For this review, take the finished solid that the model builds, in its own axes (mm). A direction names the side the tool comes from. Round coordinates to 2 decimals unless told otherwise and drop trailing zeros. Loops run counter-clockwise (first coordinate to the right, second up) from the corner with the lowest first, then second, coordinate; pieces in that order, holes last.
1. Consider section B-B on z = 43.5. State the section outline as (x, y) points.
2. Tool access review of faces 5 (the flat face through (-46, 29, -11)), 6 (the flat face through (1, 13, 32.5)), 7 (the flat face through (52, 2, 10)), 8 (the cylindrical face through (2.49, 6.48, 28.63)): name each direction out of +Z, -Z, +X, -X, +Y, -Y from which nothing blocks a thin tool from reaching the whole face with its end or side.
3. Consider section C-C on x = 43. State the section outline as (y, z) points.
4. Consider section D-D on y = 11.5. State the section outline as (x, z) points, then the cut area to 4 significant figures.
5. To check wall thickness, follow line 1 along X through (y, z) = (6.95, -28) (3 decimals); line 2 along X through (y, z) = (3.8, 43.5); line 3 along Z through (x, y) = (-41, 14). State the ranges of each line that lie inside material, in increasing order.
6. Draft analysis for pull direction Z (two halves, no side actions). For faces 1 (the flat face through (-1, 5, -46)), 2 (the flat face through (-46, 29, -4)), 3 (the cylindrical face through (56.6, 2.46, 9.14)), 4 (the flat face through (-35, 5, -28)), state which applies: released by +Z, released by -Z, zero draft, split by the parting line, or undercut.
7. Clearance check with flat-ended pins moving along their axes: pin 1 Ø10 at (x, z) = (24.5, -13.5) entering from +Y; pin 2 Ø1 at (x, z) = (3.5, 34.5) entering from +Y; pin 3 Ø2.5 at (x, z) = (-34.5, 28) entering from +Y; pin 4 Ø12 at (x, y) = (25, 29.5) entering from +Z. State where each tip first meets the part, or that it passes through.
8. Consider section A-A on y = 32.5. State the section outline as (x, z) points, then the cut area to 3 significant figures.
from build123d import *

# Parameters (mm, degrees)
BOSS_EXTRUDE1_DEPTH = 5
SKETCH2_W           = 95
SKETCH2_H           = 5
BOSS_EXTRUDE2_DEPTH = 15
SKETCH3_W           = 3
SKETCH3_H           = 75
BOSS_EXTRUDE3_DEPTH = 33
SKETCH4_R           = 2.5
SKETCH4_R_2         = 1.175
BOSS_EXTRUDE4_DEPTH = 3
CUT_EXTRUDE1_DEPTH  = 120.57529009
SKETCH6_R           = 2.2
CUT_EXTRUDE2_DEPTH  = 83.737536826
CUT_EXTRUDE3_DEPTH  = 92
FILLET1_R           = 1
FILLET2_R           = 2
BOSS_EXTRUDE5_START = -2
BOSS_EXTRUDE5_DEPTH = 16


with BuildPart() as part:
    # Sketch1 → Boss-Extrude1 (new body)
    with BuildSketch(Plane(origin=(0, 0, 0), x_dir=(1, 0, 0), z_dir=(0, 1, 0))):
        with BuildLine():
            Line((47.5, 13), (47.5, 49.5))
            Line((47.5, 49.5), (-47.5, 49.5))
            Line((-47.5, 49.5), (-47.5, -49.5))
            Line((-47.5, -49.5), (47.5, -49.5))
            Line((47.5, -49.5), (47.5, -13))
            ThreePointArc((47.5, -13), (48.378679656, -10.878679656), (50.5, -10))
            Line((50.5, -10), (54.5, -10))
            ThreePointArc((54.5, -10), (56.621320344, -9.121320344), (57.5, -7))
            Line((57.5, -7), (57.5, 7))
            ThreePointArc((57.5, 7), (56.621320344, 9.121320344), (54.5, 10))
            Line((54.5, 10), (50.5, 10))
            ThreePointArc((50.5, 10), (48.378679656, 10.878679656), (47.5, 13))
        make_face()
    extrude(amount=BOSS_EXTRUDE1_DEPTH)

    # Sketch2 → Boss-Extrude2 (add)
    with BuildSketch(Plane(origin=(0, 5, 0), x_dir=(1, 0, 0), z_dir=(0, 1, 0))):
        with Locations((0, 35)):
            Rectangle(SKETCH2_W, SKETCH2_H)
        with Locations((0, -35)):
            Rectangle(SKETCH2_W, SKETCH2_H)
    extrude(amount=BOSS_EXTRUDE2_DEPTH)

    # Sketch3 → Boss-Extrude3 (add)
    with BuildSketch(Plane(origin=(0, 5, 0), x_dir=(1, 0, 0), z_dir=(0, 1, 0))):
        with Locations((-46, 0)):
            Rectangle(SKETCH3_W, SKETCH3_H)
    extrude(amount=BOSS_EXTRUDE3_DEPTH)

    # Sketch4 → Boss-Extrude4 (add)
    # profile 1 of 4: a face of its own
    with BuildSketch(Plane(origin=(0, 5, 0), x_dir=(1, 0, 0), z_dir=(0, 1, 0))):
        with Locations(Location((-34.5, 28, 0), (0, 0, 90))):
            Circle(SKETCH4_R)
        with Locations(Location((-34.5, 28, 0), (0, 0, 270))):
            Circle(SKETCH4_R_2, mode=Mode.SUBTRACT)
    # profile 2 of 4: a face of its own
    with BuildSketch(Plane(origin=(0, 5, 0), x_dir=(1, 0, 0), z_dir=(0, 1, 0))):
        with Locations(Location((-34.5, -28, 0), (0, 0, 90))):
            Circle(SKETCH4_R)
        with Locations(Location((-34.5, -28, 0), (0, 0, 270))):
            Circle(SKETCH4_R_2, mode=Mode.SUBTRACT)
    # profile 3 of 4: a face of its own
    with BuildSketch(Plane(origin=(0, 5, 0), x_dir=(1, 0, 0), z_dir=(0, 1, 0))):
        with Locations(Location((1.5, 28, 0), (0, 0, 90))):
            Circle(SKETCH4_R)
        with Locations(Location((1.5, 28, 0), (0, 0, 270))):
            Circle(SKETCH4_R_2, mode=Mode.SUBTRACT)
    # profile 4 of 4: a face of its own
    with BuildSketch(Plane(origin=(0, 5, 0), x_dir=(1, 0, 0), z_dir=(0, 1, 0))):
        with Locations(Location((1.5, -28, 0), (0, 0, 90))):
            Circle(SKETCH4_R)
        with Locations(Location((1.5, -28, 0), (0, 0, 270))):
            Circle(SKETCH4_R_2, mode=Mode.SUBTRACT)
    extrude(amount=BOSS_EXTRUDE4_DEPTH)

    # Sketch5 → Cut-Extrude1 (cut, through all)
    with BuildSketch(Plane(origin=(-44.5, 0, 0), x_dir=(0, 0, -1), z_dir=(1, 0, 0))):
        with BuildLine():
            Line((-19, 20), (-19, 38))
            Line((-19, 38), (-11, 38))
            Line((-11, 38), (-11, 20))
            ThreePointArc((-11, 20), (-15, 16), (-19, 20))
        make_face()
        with BuildLine():
            Line((-4, 20), (-4, 38))
            Line((-4, 38), (4, 38))
            Line((4, 38), (4, 20))
            ThreePointArc((4, 20), (0, 16), (-4, 20))
        make_face()
        with BuildLine():
            Line((11, 20), (11, 38))
            Line((11, 38), (19, 38))
            Line((19, 38), (19, 20))
            ThreePointArc((19, 20), (15, 16), (11, 20))
        make_face()
    extrude(amount=-CUT_EXTRUDE1_DEPTH, mode=Mode.SUBTRACT)

    # Sketch6 → Cut-Extrude2 (cut, through all)
    with BuildSketch(Plane(origin=(0, 5, 0), x_dir=(1, 0, 0), z_dir=(0, 1, 0))):
        with Locations(Location((-35, 43.5, 0), (0, 0, 270))):
            Circle(SKETCH6_R)
        with Locations(Location((0, 43.5, 0), (0, 0, 270))):
            Circle(SKETCH6_R)
        with Locations(Location((35, 43.5, 0), (0, 0, 270))):
            Circle(SKETCH6_R)
        with Locations(Location((35, -43.5, 0), (0, 0, 90))):
            Circle(SKETCH6_R)
        with Locations(Location((0, -43.5, 0), (0, 0, 90))):
            Circle(SKETCH6_R)
        with Locations(Location((-35, -43.5, 0), (0, 0, 90))):
            Circle(SKETCH6_R)
    extrude(amount=-CUT_EXTRUDE2_DEPTH, mode=Mode.SUBTRACT)

    # Sketch7 → Cut-Extrude3 (cut)
    with BuildSketch(Plane(origin=(47.5, 0, 0), x_dir=(0, 0, -1), z_dir=(1, 0, 0))):
        Polygon((-36, 19.4), (-34, 17.4), (-37.5, 17.4), (-37.5, 20), (-36, 20), align=None)
        Polygon((37.5, 20), (37.5, 17.4), (34, 17.4), (36, 19.4), (36, 20), align=None)
    extrude(amount=-CUT_EXTRUDE3_DEPTH, mode=Mode.SUBTRACT)

    # Fillet1
    fillet1_edges = [part.edges().sort_by_distance(p)[0] for p in [
        (47.5, 2.5, -49.5),
        (47.5, 2.5, 49.5),
        (-47.5, 2.5, 49.5),
        (-47.5, 2.5, -49.5),
    ]]
    fillet(fillet1_edges, radius=FILLET1_R)

    # Fillet2
    fillet2_edges = [part.edges().sort_by_distance(p)[0] for p in [
        (0, 5, -37.5),
        (1.5, 5, 32.5),
        (0, 5, 37.5),
        (1.5, 5, -32.5),
        (-44.5, 5, 0),
    ]]
    fillet(fillet2_edges, radius=FILLET2_R - 0.0001)  # a hair under: the kernel refuses the full size

    # Sketch9 → Boss-Extrude5 (add)
    with BuildSketch(Plane.XY.offset(10).offset(BOSS_EXTRUDE5_START)):
        with BuildLine():
            Line((50.5, 5), (52, 5))
            ThreePointArc((52, 5), (51.25, 5.75), (50.5, 5))
        make_face()
    extrude(amount=-BOSS_EXTRUDE5_DEPTH)


solid = part.part
Resolved:
1. outline: (-47.5, 0) - (-37.2, 0) - (-37.2, 5) - (-47.5, 5) - close; (-32.8, 0) - (-2.2, 0) - (-2.2, 5) - (-32.8, 5) - close; (2.2, 0) - (32.8, 0) - (32.8, 5) - (2.2, 5) - close; (37.2, 0) - (47.5, 0) - (47.5, 5) - (37.2, 5) - close
2. face 5: +X, -X, +Y
2. face 6: +X, +Y
2. face 7: +Z, +X, +Y, -Y
2. face 8: +Y
3. outline: (0, -49.5) - (5, -49.5) - (5, -39.5) arc R2 cw to (7, -37.5) - (17.4, -37.5) - (17.4, -34) - (19.4, -36) - (20, -36) - (20, -32.5) - (7, -32.5) arc R2 cw to (5, -30.5) - (5, 30.5) arc R2 cw to (7, 32.5) - (20, 32.5) - (20, 36) - (19.4, 36) - (17.4, 34) - (17.4, 37.5) - (7, 37.5) arc R2 cw to (5, 39.5) - (5, 49.5) - (0, 49.5) - close
4. outline: (-47.5, -37.5) - (47.5, -37.5) - (47.5, -32.5) - (-44.5, -32.5) - (-44.5, 32.5) - (47.5, 32.5) - (47.5, 37.5) - (-47.5, 37.5) - close
4. area: 1,145 mm2
5. line 1: x = -47.5 to -44.499, -37 to -35.675, -33.325 to -32, -1 to 0.325, 2.675 to 4
5. line 2: x = -47.5 to -37.2, -32.8 to -2.2, 2.2 to 32.8, 37.2 to 47.5
5. line 3: z = -37.5 to -32.5, 32.5 to 37.5
6. face 1: zero draft
6. face 2: undercut
6. face 3: released by +Z
6. face 4: undercut
7. pin 1: stops at y = 5
7. pin 2: stops at y = 20
7. pin 3: stops at y = 8
7. pin 4: passes through
8. outline: (-47.5, -37.5) - (-44.5, -37.5) - (-44.5, -19) - (-47.5, -19) - close; (-47.5, -11) - (-44.5, -11) - (-44.5, -4) - (-47.5, -4) - close; (-47.5, 4) - (-44.5, 4) - (-44.5, 11) - (-47.5, 11) - close; (-47.5, 19) - (-44.5, 19) - (-44.5, 37.5) - (-47.5, 37.5) - close
8. area: 153 mm2
